Drawing for the job (mm, zero at the part's lowest x, y, z). Round coordinates to 2 decimals unless told otherwise and drop trailing zeros. Write each loop counter-clockwise with the first axis right and the second up, starting at its lowest first coordinate (ties: lowest second). Pieces come first, ordered by that corner, then holes. Notation, with made-up numbers: (63, 2) - (74, 2) arc R13 cw to (74, 13) - close; hole circle Ø3 at (74.25, 46.5). An arc over 180 degrees is marked (long way). Answer in a Markdown table with one row per item.
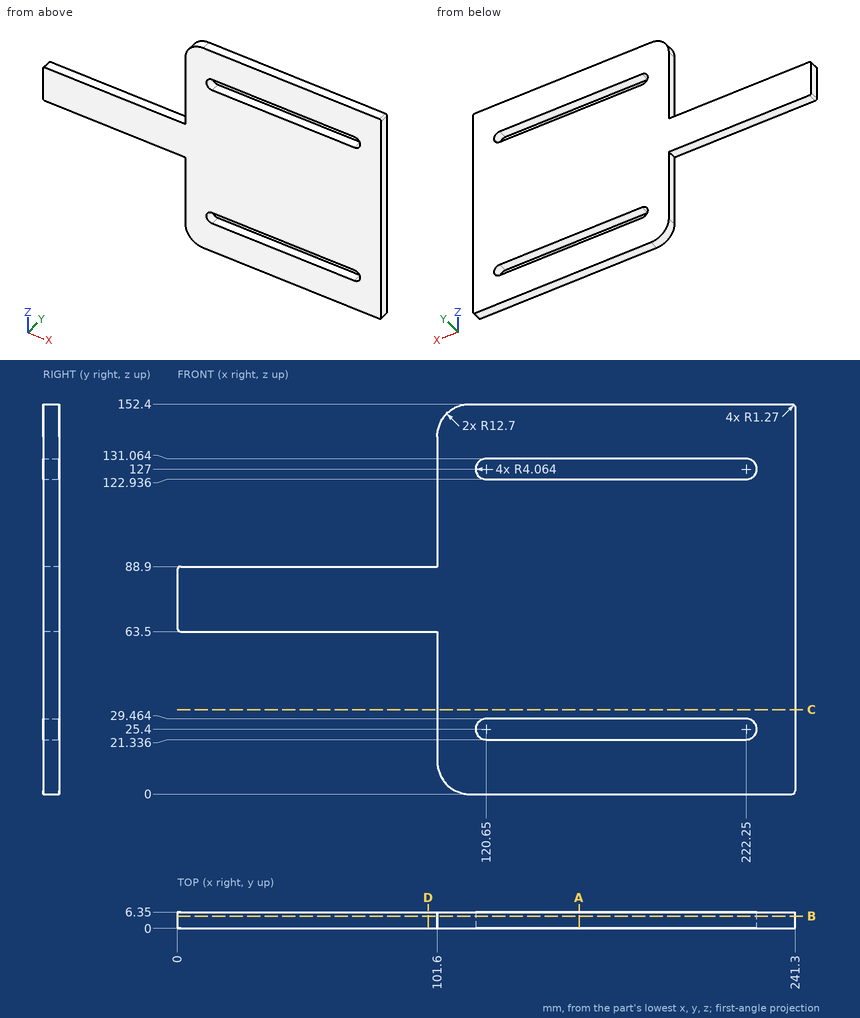
Q1. Saw through at C-C on z = 33. List the corners of the cut face in (x, y), then the cut area to 3 significant figures.
Computed:
| item | result |
|---|---|
| outline | (101.6, 0) - (241.3, 0) - (241.3, 6.35) - (101.6, 6.35) - close |
| area | 887 mm2 |
Q2. Saw through at D-D on x = 98. List the corners of the cut face in (y, z).
Computed:
| item | result |
|---|---|
| outline | (0, 63.5) - (6.35, 63.5) - (6.35, 88.9) - (0, 88.9) - close |
Q3. Drill centre lines: line 1 (Z direction, x = 126.5, y = 0.5); line 2 (Z direction, x = 93, y = 1.5); line 3 (X direction, y = 5.5, z = 58.5). Where is each one in solid material? Low to high.
Computed:
| item | result |
|---|---|
| line 1 | z = 0 to 21.34, 29.46 to 122.94, 131.06 to 152.4 |
| line 2 | z = 63.5 to 88.9 |
| line 3 | x = 101.6 to 241.3 |
Q4. Saw through at A-A on x = 157. List the corners of the cut face in (y, z).
Computed:
| item | result |
|---|---|
| outline | (0, 0) - (6.35, 0) - (6.35, 21.34) - (0, 21.34) - close; (0, 29.46) - (6.35, 29.46) - (6.35, 122.94) - (0, 122.94) - close; (0, 131.06) - (6.35, 131.06) - (6.35, 152.4) - (0, 152.4) - close |
Q5. Saw through at B-B on y = 4.75. List the corners of the cut face in (x, z).
Computed:
| item | result |
|---|---|
| outline | (0, 64.77) arc R1.27 ccw to (1.27, 63.5) - (101.6, 63.5) - (101.6, 12.7) arc R12.7 ccw to (114.3, 0) - (240.03, 0) arc R1.27 ccw to (241.3, 1.27) - (241.3, 151.13) arc R1.27 ccw to (240.03, 152.4) - (114.3, 152.4) arc R12.7 ccw to (101.6, 139.7) - (101.6, 88.9) - (1.27, 88.9) arc R1.27 ccw to (0, 87.63) - close; hole (120.65, 21.34) - (222.25, 21.34) arc R4.06 ccw to (222.25, 29.46) - (120.65, 29.46) arc R4.06 ccw to start; hole (120.65, 122.94) - (222.25, 122.94) arc R4.06 ccw to (222.25, 131.06) - (120.65, 131.06) arc R4.06 ccw to start |
Q6. Flat gauge pins, fed straight in: pin 1 (3 mm diameter, centred on x = 168, y = 3, fed in from -Z); pin 2 (3 mm diameter, centred on y = 3.5, z = 32.5, fed in from -X). Where does each tip first touch, or does it go through?
Computed:
| item | result |
|---|---|
| pin 1 | stops at z = 0 |
| pin 2 | stops at x = 101.6 |
